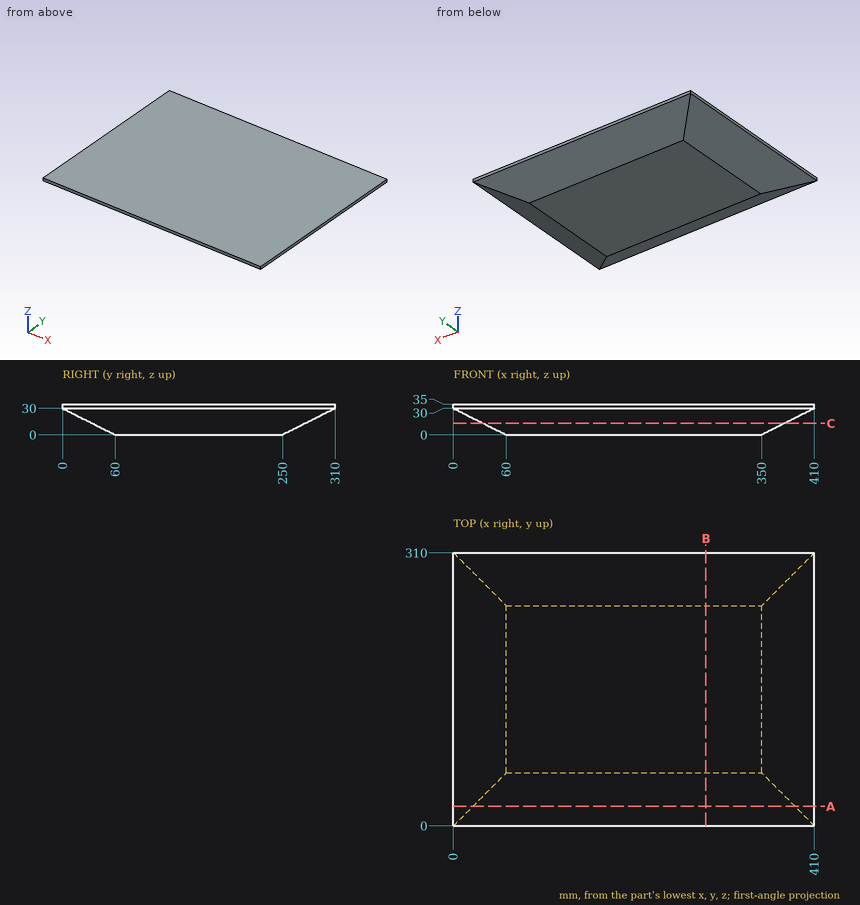
The drawing under review shows one solid part. Ordinate dimensions are in mm from its lowest x, y, z. Round coordinates to 2 decimals unless told otherwise and drop trailing zeros. Write each loop counter-clockwise with the first axis right and the second up, starting at its lowest first coordinate (ties: lowest second). Pieces come first, ordered by that corner, then holes. Notation, with made-up numbers: (68, -20.75) -> (117, -20.75) arc R23 ccw to (117, -8.75) -> close; hole circle Ø7 at (-27, -14.5). An arc over 180 degrees is marked (long way). One line per question, with ' | ' between items. Start each with the question number.
(1) Insertion check: P1, Ø10, axis at x = 179, z = 14.5, coming from the +Y side; P2, Ø3, axis at y = 105.5, z = 6, coming from the +X side; P3, Ø2, axis at y = 75, z = 23, coming from the +X side. Each pin has a flat end and moves straight along its axis. Give the tip position at first contact, or say it passes through.
(2) Add section A-A, the plane y = 22. Write out the cut boundary in (x, z), plus the area to 3 significant figures.
(3) Add section B-B, the plane x = 286.5. Write out the cut boundary in (y, z), plus the area to 3 significant figures.
(4) For line 1 along X through (y, z) = (163.5, 7.5); line 2 along X through (y, z) = (27, 25.5); line 3 along Y through (x, z) = (73, 13), list the stretches that pass through material, from the lowest coordinate up. Write a range as from..to.
(5) Add section C-C, the plane z = 13. Write out the cut boundary in (x, y), plus the area to 3 significant figures.
Answer list:
1) P1: y = 289 | P2: x = 365 | P3: x = 398
2) outline: (0, 30) -> (22, 19) -> (388, 19) -> (410, 30) -> (410, 35) -> (0, 35) -> close | area: 6,320 mm²
3) outline: (0, 30) -> (60, 0) -> (250, 0) -> (310, 30) -> (310, 35) -> (0, 35) -> close | area: 9,050 mm²
4) line 1: 45..365 | line 2: 9..401 | line 3: 34..276
5) outline: (34, 34) -> (376, 34) -> (376, 276) -> (34, 276) -> close | area: 82,800 mm²
